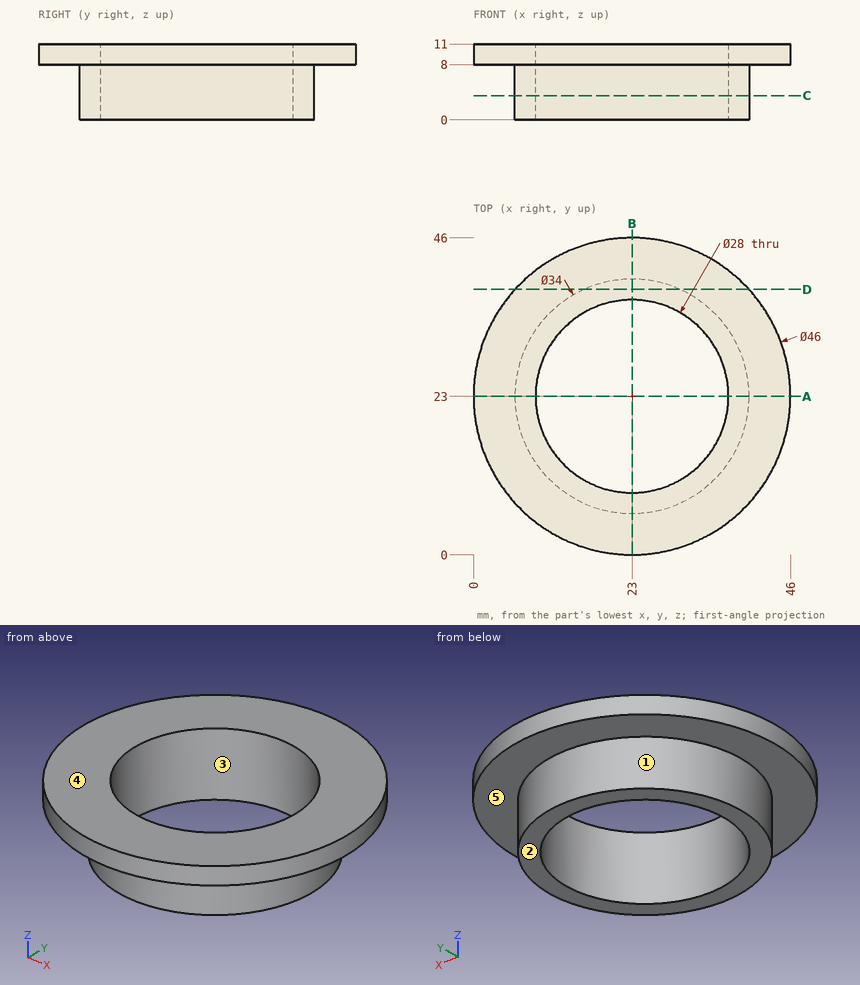
Can you work these out from the drawing? Everything is in mm from the part's minimum corner. A direction names the side the tool comes from. Round coordinates to 2 decimals unless told otherwise and drop trailing zeros. Order: outer loops, then holes, each group sorted by start corner. A loop starts at its lowest first (then second) coordinate and runs counter-clockwise, first axis right, second up. Notation, with made-up numbers: (-19, 67) - (-5, 67) arc R20 ccw to (-5, 89) - close; hole circle Ø5 at (-23, -27.75). An arc over 180 degrees is marked (long way). Answer in a Markdown table with one row per item.
(1) If we mould it in two halves opening along Y, with no side actions, what happens to the marked faces 1, 2 and 3? For each: released by +Y, released by -Y, zero draft, split by the parting line, or undercut.
From the geometry:
| item | result |
|---|---|
| face 1 | split by the parting line |
| face 2 | zero draft |
| face 3 | undercut |
(2) Which directions (+Z, -Z, +X, -X, +Y, -Y) give clear straight access to the entire face, cutting with the end or side of a thin tool? Please do the marked faces 4 and 5.
From the geometry:
| item | result |
|---|---|
| face 4 | +Z, +X, -X, +Y, -Y |
| face 5 | -Z |
(3) Please list where these lines run through material, in increasing order: L1, parallel to Y at x = 23, z = 5.25; L2, parallel to Z at x = 37.5, y = 10.5; L3, parallel to X at y = 25.5, z = 5.75. Write a range as from..to.
From the geometry:
| item | result |
|---|---|
| L1 | y = 6..9, 37..40 |
| L2 | z = 8..11 |
| L3 | x = 6.18..9.23, 36.77..39.82 |
(4) Suppose I cut it at D-D, the plane y = 38.5. Please give me the cut outline in (x, z), plus the area to 3 significant figures.
From the geometry:
| item | result |
|---|---|
| outline | (6.01, 8) - (16.02, 8) - (16.02, 0) - (29.98, 0) - (29.98, 8) - (39.99, 8) - (39.99, 11) - (6.01, 11) - close |
| area | 214 mm2 |
(5) Suppose I cut it at C-C, the plane z = 3.5. Please give me the cut outline in (x, y).
From the geometry:
| item | result |
|---|---|
| outline | circle Ø34 at (23, 23); hole circle Ø28 at (23, 23) |
(6) For P1, Ø3, axis at x = 23, z = 4.5, coming from the -Y side; P2, Ø4, axis at x = 31, z = 5.5, coming from the -Y side; P3, Ø3, axis at x = 21.5, z = 7.5, coming from the -Y side, each with a flat end and sliding along its axis, tell me the tip position at first contact or that it passes through.
From the geometry:
| item | result |
|---|---|
| P1 | stops at y = 6 |
| P2 | stops at y = 7.09 |
| P3 | stops at y = 0 |
(7) Suppose I cut it at A-A, the plane y = 23. Please give me the cut outline in (x, z).
From the geometry:
| item | result |
|---|---|
| outline | (0, 8) - (6, 8) - (6, 0) - (9, 0) - (9, 11) - (0, 11) - close; (37, 0) - (40, 0) - (40, 8) - (46, 8) - (46, 11) - (37, 11) - close |
